```python
from build123d import *

# Parameters (mm, degrees)
ESQUISSE1_W             = 2
ESQUISSE1_H             = 37
ESQUISSE1_W_2           = 24
BOSS_EXTRU_1_DEPTH      = 30
ENL_V_MAT_EXTRU_3_DEPTH = 40
CONG_1_R                = 0.5
ESQUISSE4_R             = 0.34
ENL_V_MAT_EXTRU_4_DEPTH = 12
ESQUISSE5_R             = 1.5
ENL_V_MAT_EXTRU_6_DEPTH = 16


with BuildPart() as part:
    # Esquisse1 → Boss.-Extru.1 (new body)
    with BuildSketch(Plane(origin=(0, 0, 0), x_dir=(1, 0, 0), z_dir=(0, 1, 0))):
        with Locations((-13, 0)):
            Rectangle(ESQUISSE1_W, ESQUISSE1_H)
        Rectangle(ESQUISSE1_W_2, ESQUISSE1_H)
        with Locations((13, 0)):
            Rectangle(ESQUISSE1_W, ESQUISSE1_H)
    extrude(amount=BOSS_EXTRU_1_DEPTH)

    # Esquisse3 → Enlèv. mat.-Extru.3 (cut)
    with BuildSketch(Plane(origin=(0, 0, -18.5), x_dir=(-1, 0, 0), z_dir=(0, 0, -1))):
        Polygon((-8, 15), (8, 15), (14, 30), (-14, 30), align=None)
    extrude(amount=-ENL_V_MAT_EXTRU_3_DEPTH, mode=Mode.SUBTRACT)

    # Congé1
    cong_1_edges = [part.edges().sort_by_distance(p)[0] for p in [
        (14, 30, 0),
        (-14, 30, 0),
    ]]
    fillet(cong_1_edges, radius=CONG_1_R)

    # Esquisse4 → Enlèv. mat.-Extru.4 (cut)
    with BuildSketch(Plane(origin=(0, 15, 0), x_dir=(1, 0, 0), z_dir=(0, 1, 0))):
        with Locations(Location((0, 8.5, 0), (0, 0, 180))):
            Circle(ESQUISSE4_R)
        with Locations(Location((0, -8.5, 0), (0, 0, 180))):
            Circle(ESQUISSE4_R)
    extrude(amount=-ENL_V_MAT_EXTRU_4_DEPTH, mode=Mode.SUBTRACT)

    # Esquisse5 → Enlèv. mat.-Extru.6 (cut)
    with BuildSketch(Plane.ZY.offset(14)):
        with Locations((-8.5, 3)):
            Circle(ESQUISSE5_R)
        with Locations((8.5, 3)):
            Circle(ESQUISSE5_R)
    extrude(amount=-ENL_V_MAT_EXTRU_6_DEPTH, mode=Mode.SUBTRACT)


solid = part.part
```
CAD build for the part. Positions are in the model's coordinates, mm. A direction names the side the tool comes from. Round coordinates to 2 decimals unless told otherwise and drop trailing zeros. Order: outer loops, then holes, each group sorted by start corner. A loop starts at its lowest first (then second) coordinate and runs counter-clockwise, first axis right, second up. Notation, with made-up numbers: (27.25, -36) -> (80.25, -36) arc R8 cw to (80.25, -26) -> close; hole circle Ø1 at (63.5, 29.5). An arc over 180 degrees is marked (long way). One line per question, with ' | ' between items.
Q1. Slice it at B-B (z = -10.5). Write the cut outline in (x, y), then the cut area to 3 significant figures.
Completed:
outline: (-14, 0) -> (14, 0) -> (14, 27.4) arc R0.5 ccw to (13.04, 27.59) -> (8, 15) -> (-8, 15) -> (-13.04, 27.59) arc R0.5 ccw to (-14, 27.4) -> close | area: 508 mm^2
Q2. Drop flat-ended pins along their axis: pin 1 (10 mm diameter, centred on x = 5, z = 9.5, fed in from +Y); pin 2 (2.5 mm diameter, centred on y = 3, z = -8.5, fed in from -X); pin 3 (6 mm diameter, centred on x = -5.5, z = -4.5, fed in from +Y). Give the stop position or say it passes through.
Completed:
pin 1: stops at y = 20 | pin 2: stops at x = 2 | pin 3: stops at y = 16.25
Q3. Which spindle directions (+Z, -Z, +X, -X, +Y, -Y) get a long thin tool onto all of the face, cutting with end or side? Do faces 4 (the flat face through (-10.483, 21.207, -0.259)), 5 (the cylindrical face through (-6.1, 2.1, -9.7)), 6 (the flat face through (-14, 14, 0)). Say none if no direction does.
Completed:
face 4: +Z, -Z, +Y | face 5: -X | face 6: +Z, -Z, -X, +Y, -Y
Q4. Slice it at D-D (y = 3). Write the cut outline in (x, z).
Completed:
outline: (-14, -18.5) -> (14, -18.5) -> (14, 18.5) -> (-14, 18.5) -> (-14, 10) -> (2, 10) -> (2, 7) -> (-14, 7) -> (-14, -7) -> (2, -7) -> (2, -10) -> (-14, -10) -> close
Q5. Slice it at A-A (y = 17.5). Write the cut outline in (x, z).
Completed:
outline: (-14, -18.5) -> (-9, -18.5) -> (-9, 18.5) -> (-14, 18.5) -> close; (9, -18.5) -> (14, -18.5) -> (14, 18.5) -> (9, 18.5) -> close
Q6. Slice it at C-C (x = -10.75). Write the cut outline in (y, z) (3 decimals), then the cut area to 3 significant figures.
Completed:
outline: (0, -18.5) -> (21.875, -18.5) -> (21.875, 18.5) -> (0, 18.5) -> close; hole circle Ø3 at (3, -8.5); hole circle Ø3 at (3, 8.5) | area: 795 mm^2
Q7. Probe probe 1 along Z at (x, y) = (0, 7.25); probe 2 along X at (y, z) = (12.75, -8.5); probe 3 along Y at (x, z) = (2.75, -12.5). List the from-to ranges inside material, lowest first.
Completed:
probe 1: z = -18.5 to -8.84, -8.16 to 8.16, 8.84 to 18.5 | probe 2: x = -14 to -0.34, 0.34 to 14 | probe 3: y = 0 to 15
Q8. Two-plate mould, pull along Z, no slides. Class faces 1 (the flat face through (0, 11, -18.5)), 2 (the flat face through (10.55, 21.38, -0.26)), 3 (the flat face through (2, 3, 8)): released by +Z, released by -Z, zero draft, split by the parting line, or undercut.
Completed:
face 1: released by -Z | face 2: zero draft | face 3: undercut
